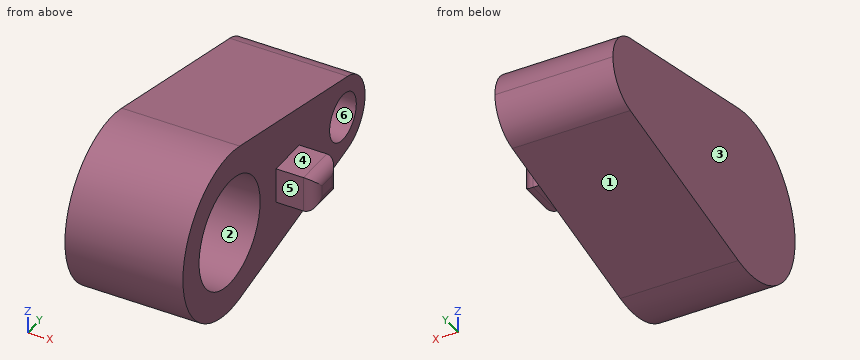
```python
from build123d import *

# Parameters (mm, degrees)
F1_DEPTH = 76.2
F2_R     = 35.044317
F3_DEPTH = 50.8
F4_R     = 15.315164
F5_DEPTH = 50.8
F6_W     = 26.776026
F6_H     = 22.917912
F7_DEPTH = 25.4
F8_R     = 7.62


with BuildPart() as f1:
    # F0 (on Right) → F1 (new body)
    with BuildSketch(Plane.YZ):
        with BuildLine():
            ThreePointArc((-54.972521, -52.316467), (-24.786857, -33.537675), (-12.995266, 0))
            ThreePointArc((-12.995266, 0), (-24.786857, 33.537675), (-54.972521, 52.316467))
            ThreePointArc((-54.972521, 52.316467), (-120.174799, 0), (-54.972521, -52.316467))
        make_face()
        with BuildLine():
            ThreePointArc((-54.972521, 52.316467), (-24.786857, 33.537675), (-12.995266, 0))
            ThreePointArc((-12.995266, 0), (-24.786857, -33.537675), (-54.972521, -52.316467))
            Line((-54.972521, -52.316467), (69.009942, -24.796493))
            ThreePointArc((69.009942, -24.796493), (38.105947, 0), (69.009942, 24.796493))
            Line((69.009942, 24.796493), (-54.972521, 52.316467))
        make_face()
        with BuildLine():
            ThreePointArc((88.905947, 0), (83.317074, 15.895888), (69.009942, 24.796493))
            ThreePointArc((69.009942, 24.796493), (38.105947, 0), (69.009942, -24.796493))
            ThreePointArc((69.009942, -24.796493), (83.317074, -15.895888), (88.905947, 0))
        make_face()
    extrude(amount=F1_DEPTH)

    # F2 (on face) → F3 (cut)
    with BuildSketch(Plane.YZ.offset(76.2)):
        with Locations((-66.585032, 0)):
            Circle(F2_R)
    extrude(amount=-F3_DEPTH, mode=Mode.SUBTRACT)

    # F4 (on face) → F5 (cut)
    with BuildSketch(Plane.YZ.offset(76.2)):
        with Locations((63.536301, 0)):
            Circle(F4_R)
    extrude(amount=-F5_DEPTH, mode=Mode.SUBTRACT)

    # F6 (on face) → F7 (join)
    with BuildSketch(Plane.YZ.offset(76.2)):
        Rectangle(F6_W, F6_H)
    extrude(amount=F7_DEPTH)

    # F8
    f8_edges = [f1.edges().sort_by_distance(p)[0] for p in [
        (101.6, -13.388013, 0),
        (101.6, 0, -11.458956),
        (101.6, 13.388013, 0),
        (101.6, 0, 11.458956),
    ]]
    fillet(f8_edges, radius=F8_R)


solid = f1.part
```
The listing builds one solid part. Answer for the finished solid, in the listing's coordinates (mm). Face numbers are marked on the shaded views. A direction names the side the tool comes from. Coordinates: 2 decimals unless noted, no trailing zeros. Loops run counter-clockwise (first coordinate to the right, second up) from the corner with the lowest first, then second, coordinate; pieces in that order, holes last. Notation, with made-up numbers: (28, 77) - (81, 77) arc R16 cw to (81, 100) - close; hole circle Ø11 at (88, 80.25). An arc over 180 degrees is marked (long way). Use a Markdown table: item, result. Add a question column.
1) The part is cut by section B-B, the plane y = 64. Give the vertices of the cut face in (x, z), and give its area (3 significant figures).
2) The part is cut by section A-A, the plane x = 59.5. Give the vertices of the cut face in (y, z), and give its area (3 significant figures).
3) For the marked faces 4, 5 and 6, determine the directions among +Z, -Z, +X, -X, +Y, -Y from which every point of the face is accessible in a straight line to the end or side of a thin tool.
4) The mould has two halves that part along Y. Classify the marked faces 1, 2 and 3: released by +Y, released by -Y, zero draft, split by the parting line, or undercut.
5) The part is cut by section D-D, the plane x = 81. Give the vertices of the cut face in (y, z), and give its area (3 significant figures).
6) The part is cut by section C-C, the plane z = -19.5. Give the vertices of the cut face in (x, y).
7) Given pin 1 (8 mm diameter, centred on x = 16.5, z = -16.5, fed in from -Y); pin 2 (2 mm diameter, centred on x = 57.5, z = -33.5, fed in from -Y); pin 3 (9 mm diameter, centred on x = 83.5, y = 4, fed in from -Z), each flat-ended and moving along its own axis, determine where each tip first touches the part or whether it passes through.
8) Find the intervals of material crossed by line 1 (X direction, y = -78.5, z = -33); line 2 (Y direction, x = 74, z = 6); line 3 (Z direction, x = 79, y = 2), in increasing order.
Here are the results:
| question | item | result |
|---|---|---|
| 1 | outline | (0, -25.91) - (76.2, -25.91) - (76.2, -15.31) - (25.4, -15.31) - (25.4, 15.31) - (76.2, 15.31) - (76.2, 25.91) - (0, 25.91) - close |
| 1 | area | 2,390 mm^2 |
| 2 | outline | (-54.97, -52.32) - (69.01, -24.8) arc R25.4 ccw to (69.01, 24.8) - (-54.97, 52.32) arc R53.59 ccw (long way) to start; hole circle Ø70.09 at (-66.59, 0); hole circle Ø30.63 at (63.54, 0) |
| 2 | area | 11,400 mm^2 |
| 3 | face 4 | +Z, +X, +Y, -Y |
| 3 | face 5 | +Z, -Z, +X, -Y |
| 3 | face 6 | +X |
| 4 | face 1 | released by +Y |
| 4 | face 2 | undercut |
| 4 | face 3 | zero draft |
| 5 | outline | (-13.39, -11.46) - (13.39, -11.46) - (13.39, 11.46) - (-13.39, 11.46) - close |
| 5 | area | 614 mm^2 |
| 6 | outline | (0, -116.5) - (76.2, -116.5) - (76.2, -95.7) - (25.4, -95.7) - (25.4, -37.47) - (76.2, -37.47) - (76.2, 79.78) - (0, 79.78) - close |
| 7 | pin 1 | stops at y = -118.7 |
| 7 | pin 2 | stops at y = -109.2 |
| 7 | pin 3 | stops at z = -11.46 |
| 8 | line 1 | x = 0 to 76.2 |
| 8 | line 2 | y = -119.84 to -101.11, -32.06 to 49.45, 77.63 to 88.19 |
| 8 | line 3 | z = -11.46 to 11.46 |
